Check sheet for the modelled part. Datum: model origin and axes. Units: mm. A direction names the side the tool comes from. Coordinates: 2 decimals unless noted, no trailing zeros. Write each loop counter-clockwise with the first axis right and the second up, starting at its lowest first coordinate (ties: lowest second). Pieces come first, ordered by that corner, then holes. Notation, with made-up numbers: M 13,-22 L 54,-22 A29 ccw 54,-2 Z; hole C 48,-36.5 d10. An arc over 180 degrees is marked long. Answer as CSV lines item,"result". Start each with the question number.
1) Section check B-B (x = 0). Record the cut outline in (y, z) (3 decimals), and give its area (3 significant figures).
2) Material ranges on L1, parallel to Z at x = 0, y = -34.5; L2, parallel to Z at x = 0, y = -192.75; L3, parallel to X at y = -163.5, z = -17.5, recorded low to high. Write a range as [from, to].
3) Access from +Z, -Z, +X, -X, +Y, -Y to the whole of each face (thin tool, end or side, straight path). Record for faces 4 (the flat face through (-16, -170.967, 35)), 5 (the flat face through (16, 170.967, 35)), 6 (the flat face through (-1, -200.025, -44)).
4) Section check A-A (z = 0). Record the cut outline in (x, y) (3 decimals).
5) Draft check along X on faces 1 (the conical face through (-14.652, 199.871, -65.984)), 2 (the flat face through (-1, 200.025, -44)), 3 (the cylindrical face through (40.538, -185.7, 12.766)). Enter one of: +X half, -X half, draft (parallel to the pull), parting line (faces both ways), or undercut.
6) Go/stop test with flat-tipped pins: pin 1 Ø6 at (x, y) = (-26, 159.5) entering from -Z; pin 2 Ø12 at (y, z) = (-66.5, -2) entering from -X; pin 3 Ø6 at (y, z) = (14.5, 23) entering from +X; pin 4 Ø1 at (x, y) = (39, 86.5) entering from +Z. Record where each tip stops, or that it passes through.
7) Section check C-C (y = 10.5). Record the cut outline in (x, z), and give its area (3 significant figures).
from build123d import *

# Parameters (mm, degrees)
F0_R           = 70.612
F1_DEPTH       = 200.025
F2_SIZE        = 3.175
F4_D           = 76.2
F4_CBORE_D     = 85.0011
F4_CBORE_DEPTH = 29.0576
F5_R           = 42.50055
F6_DEPTH       = 29.0576


with BuildPart() as f1:
    # F0 (on Front) → F1 (new body, symmetric)
    with BuildSketch(Plane.XZ):
        Circle(F0_R)
    extrude(amount=F1_DEPTH, both=True)

    # F2
    f2_edges = [f1.edges().sort_by_distance(p)[0] for p in [
        (-70.612, -200.025, 0),
        (-70.612, 200.025, 0),
    ]]
    chamfer(f2_edges, length=F2_SIZE)

    # F4 (through all)
    with Locations(Plane(origin=(0, 200.025, 0), x_dir=(-1, 0, 0), z_dir=(0, 1, 0))):
        with Locations((0, 0)):
            CounterBoreHole(F4_D / 2, F4_CBORE_D / 2, F4_CBORE_DEPTH)

    # F5 (on face) → F6 (cut)
    with BuildSketch(Plane.XZ.offset(200.025)):
        Circle(F5_R)
    extrude(amount=-F6_DEPTH, mode=Mode.SUBTRACT)


solid = f1.part
Results found:
1,outline,"M -200.025,-67.437 L -196.85,-70.612 L 196.85,-70.612 L 200.025,-67.437 L 200.025,-42.501 L 170.967,-42.501 L 170.967,-38.1 L -170.967,-38.1 L -170.967,-42.501 L -200.025,-42.501 Z; M -200.025,42.501 L -170.967,42.501 L -170.967,38.1 L 170.967,38.1 L 170.967,42.501 L 200.025,42.501 L 200.025,67.437 L 196.85,70.612 L -196.85,70.612 L -200.025,67.437 Z"
1,area,"25,500 mm2"
2,L1,"z = [-70.61, -38.1], [38.1, 70.61]"
2,L2,"z = [-70.61, -42.5], [42.5, 70.61]"
2,L3,"x = [-68.41, -33.84], [33.84, 68.41]"
3,face 4,"-Y"
3,face 5,"+Y"
3,face 6,"+Z, -Z, +X, -X, -Y"
4,outline,"M -70.612,-196.85 L -67.437,-200.025 L -42.501,-200.025 L -42.501,-170.967 L -38.1,-170.967 L -38.1,170.967 L -42.501,170.967 L -42.501,200.025 L -67.437,200.025 L -70.612,196.85 Z; M 38.1,-170.967 L 42.501,-170.967 L 42.501,-200.025 L 67.437,-200.025 L 70.612,-196.85 L 70.612,196.85 L 67.437,200.025 L 42.501,200.025 L 42.501,170.967 L 38.1,170.967 Z"
5,face 1,"parting line"
5,face 2,"draft"
5,face 3,"undercut"
6,pin 1,"stops at z = -66.76"
6,pin 2,"stops at x = -70.61"
6,pin 3,"stops at x = 67.72"
6,pin 4,"stops at z = 59.19"
7,outline,"C 0,0 d141.22; hole C 0,0 d76.2"
7,area,"11,100 mm2"
